from build123d import *

# Parameters (mm, degrees)
SKETCH1_W           = 50
SKETCH1_H           = 50
SKETCH1_R           = 2.75
BOSS_EXTRUDE1_DEPTH = 20
FILLET1_R           = 3
SKETCH2_R           = 1.4
CUT_EXTRUDE1_DEPTH  = 8


with BuildPart() as part:
    # Sketch1 → Boss-Extrude1 (new body)
    with BuildSketch(Plane(origin=(0, 0, 0), x_dir=(1, 0, 0), z_dir=(0, 1, 0))):
        with Locations((-3, 0)):
            Rectangle(SKETCH1_W, SKETCH1_H)
        with Locations(Location((-15, 20, 0), (0, 0, 270))):
            Circle(SKETCH1_R, mode=Mode.SUBTRACT)
        with Locations(Location((15, 20, 0), (0, 0, 270))):
            Circle(SKETCH1_R, mode=Mode.SUBTRACT)
        with Locations(Location((-15, -20, 0), (0, 0, 270))):
            Circle(SKETCH1_R, mode=Mode.SUBTRACT)
        with Locations(Location((15, -20, 0), (0, 0, 270))):
            Circle(SKETCH1_R, mode=Mode.SUBTRACT)
    extrude(amount=BOSS_EXTRUDE1_DEPTH)

    # Fillet1
    fillet1_edges = [part.edges().sort_by_distance(p)[0] for p in [
        (22, 10, 25),
        (22, 10, -25),
    ]]
    fillet(fillet1_edges, radius=FILLET1_R)

    # Sketch2 → Cut-Extrude1 (cut)
    with BuildSketch(Plane.ZY.offset(28)):
        with Locations((-19, 14)):
            Circle(SKETCH2_R)
        with Locations((0, 4)):
            Circle(SKETCH2_R)
        with Locations((19, 14)):
            Circle(SKETCH2_R)
    extrude(amount=-CUT_EXTRUDE1_DEPTH, mode=Mode.SUBTRACT)


solid = part.part
Read the model definition and answer for the solid it produces. Units are mm, in the model's axes. A direction names the side the tool comes from. Coordinates: 2 decimals unless noted, no trailing zeros. Loops run counter-clockwise (first coordinate to the right, second up) from the corner with the lowest first, then second, coordinate; pieces in that order, holes last.
Q1. Each of these flat-tipped pins is pushed along its axis until it touches: pin 1 Ø3.5 at (x, z) = (15, 20) entering from +Y; pin 2 Ø2.5 at (y, z) = (14, -19) entering from -X. Where does it stop, or does it pass through?
Q2. Consider probe 1 along X at (y, z) = (7.75, 20); probe 2 along X at (y, z) = (9.5, -18.5); probe 3 along Z at (x, y) = (16, 3.5). Determine where each line is inside the solid, lowest interval first.
Q3. The part is cut by section C-C on z = 19. Write down the section's boundary in (x, y), and give its area (3 significant figures).
Q4. Which of the six approach directions +Z, -Z, +X, -X, +Y, -Y give full straight-line access (tool end or side, diameter ignored) to faces 5 (the face through (15.121, 9.86, -22.747)), 6 (the face through (-24.06, 14.95, 17.97))?
Q5. The part is cut by section B-B on y = 7. Write down the section's boundary in (x, z), and give its area (3 significant figures).
Q6. The part is cut by section A-A on x = 15. Write down the section's boundary in (y, z).
Q7. The part is cut by section D-D on z = 0. Write down the section's boundary in (x, y), and give its area (3 significant figures).
Q8. The mould has two halves that part along Z. Classify faces 1 (the face through (21.1, 10.14, 24.14)), 2 (the face through (-5, 10, -25)), 3 (the face through (-20, 14, -19)), 4 (the face through (-3, 20, 0)): +Z half, -Z half, draft (parallel to the pull), parting line (faces both ways), or undercut.
Results below:
1. pin 1: passes through
1. pin 2: stops at x = -20
2. probe 1: x = -28 to -17.75, -12.25 to 12.25, 17.75 to 22
2. probe 2: x = -28 to -17.3, -12.7 to 12.7, 17.3 to 22
2. probe 3: z = -25 to -22.56, -17.44 to 17.44, 22.56 to 25
3. outline: (-28, 0) - (-17.56, 0) - (-17.56, 20) - (-28, 20) - (-28, 15.4) - (-20, 15.4) - (-20, 12.6) - (-28, 12.6) - close; (-12.44, 0) - (12.44, 0) - (12.44, 20) - (-12.44, 20) - close; (17.56, 0) - (22, 0) - (22, 20) - (17.56, 20) - close
3. area: 773 mm2
4. face 5: +Y, -Y
4. face 6: -X
5. outline: (-28, -25) - (19, -25) arc R3 ccw to (22, -22) - (22, 22) arc R3 ccw to (19, 25) - (-28, 25) - close; hole circle Ø5.5 at (-15, -20); hole circle Ø5.5 at (-15, 20); hole circle Ø5.5 at (15, -20); hole circle Ø5.5 at (15, 20)
5. area: 2,400 mm2
6. outline: (0, -25) - (20, -25) - (20, -22.75) - (0, -22.75) - close; (0, -17.25) - (20, -17.25) - (20, 17.25) - (0, 17.25) - close; (0, 22.75) - (20, 22.75) - (20, 25) - (0, 25) - close
7. outline: (-28, 0) - (22, 0) - (22, 20) - (-28, 20) - (-28, 5.4) - (-20, 5.4) - (-20, 2.6) - (-28, 2.6) - close
7. area: 978 mm2
8. face 1: +Z half
8. face 2: -Z half
8. face 3: undercut
8. face 4: draft
